```python
from build123d import *

# Parameters (mm, degrees)
ESQUISSE1_R                  = 11.15
BOSS_EXTRU_1_DEPTH           = 2
BOSS_EXTRU_2_DEPTH           = 80
BOSS_EXTRU_3_DEPTH           = 2.3
ENL_V_MAT_EXTRU_1_DEPTH      = 106.452595985
ENL_V_MAT_EXTRU_1_DEPTH_BACK = 106.452595985
ESQUISSE4_R                  = 1.55
BOSS_EXTRU_4_DEPTH           = 2
ENL_V_MAT_EXTRU_2_DEPTH      = 10
CONG_1_R                     = 2


with BuildPart() as part:
    # Esquisse1 → Boss.-Extru.1 (new body)
    with BuildSketch(Plane.XY):
        Polygon((-24.325901808, 28), (24.325901808, 28), (28, 24.325901808), (28, -24.325901808), (24.325901808, -28), (-24.325901808, -28), (-28, -24.325901808), (-28, 24.325901808), align=None)
        Circle(ESQUISSE1_R, mode=Mode.SUBTRACT)
    extrude(amount=BOSS_EXTRU_1_DEPTH)

    # Esquisse2 → Boss.-Extru.2 (add)
    with BuildSketch(Plane.XY.offset(2)):
        Polygon((-28, 24.325901808), (-28, -24.325901808), (-24.325901808, -28), (24.325901808, -28), (28, -24.325901808), (28, 24.325901808), (24.325901808, 28), (-24.325901808, 28), align=None)
        Polygon((-26.5, 23.704581464), (-26.5, -23.704581464), (-23.704581464, -26.5), (23.704581464, -26.5), (26.5, -23.704581464), (26.5, 23.704581464), (23.704581464, 26.5), (-23.704581464, 26.5), align=None, mode=Mode.SUBTRACT)
    extrude(amount=BOSS_EXTRU_2_DEPTH)

    # Esquisse3 → Boss.-Extru.3 (add)
    with BuildSketch(Plane(origin=(0, 0, 0), x_dir=(-1, 0, 0), z_dir=(0, 0, -1))):
        Polygon((-28, -20), (-28, 20), (-35.5, 12.5), (-35.5, -12.5), align=None)
        Polygon((-31.75, 3.175426481), (-34.5, 1.58771324), (-34.5, -1.58771324), (-31.75, -3.175426481), (-29, -1.58771324), (-29, 1.58771324), align=None, mode=Mode.SUBTRACT)
    extrude(amount=-BOSS_EXTRU_3_DEPTH)

    # Esquisse4 → Enlèv. mat.-Extru.1 (cut, two sides: drawn at the far end of the back side and taken through both)
    with BuildSketch(Plane(origin=(0, 28, 0), x_dir=(1, 0, 0), z_dir=(0, 1, 0)).offset(-ENL_V_MAT_EXTRU_1_DEPTH_BACK)):
        with Locations((0, -76)):
            Circle(ESQUISSE4_R)
    extrude(amount=ENL_V_MAT_EXTRU_1_DEPTH + ENL_V_MAT_EXTRU_1_DEPTH_BACK, mode=Mode.SUBTRACT)

    # Esquisse5 → Boss.-Extru.4 (add)
    with BuildSketch(Plane.XY.offset(2)):
        Polygon((-10.828088474, -1.05), (-12.1, -1.05), (-12.1, 1.05), (-10.828088474, 1.05), (-9.6, 1.05), (-9.6, -1.05), align=None)
    extrude(amount=-BOSS_EXTRU_4_DEPTH)

    # Esquisse6 → Enlèv. mat.-Extru.2 (cut)
    with BuildSketch(Plane.XY.offset(2.3)):
        Polygon((28, -20), (35.5, -12.5), (35.5, 12.5), (28, 20), align=None)
    extrude(amount=-ENL_V_MAT_EXTRU_2_DEPTH, mode=Mode.SUBTRACT)

    # Congé1
    cong_1_edges = [part.edges().sort_by_distance(p)[0] for p in [
        (-23.704581464, -26.5, 42),
        (23.704581464, -26.5, 42),
        (26.5, -23.704581464, 42),
        (26.5, 23.704581464, 42),
        (23.704581464, 26.5, 42),
        (-23.704581464, 26.5, 42),
        (-26.5, 23.704581464, 42),
        (-26.5, -23.704581464, 42),
    ]]
    fillet(cong_1_edges, radius=CONG_1_R)


solid = part.part
```
Work out the finished part from the listing and answer in its coordinate system (mm). A direction names the side the tool comes from. Give positions to 0.01 mm unless a question says otherwise; leave off trailing zeros. Loops run counter-clockwise (first coordinate to the right, second up) from the corner with the lowest first, then second, coordinate; pieces in that order, holes last. Notation, with made-up numbers: (33.25, 75.5) -> (44.25, 75.5) arc R18 ccw to (44.25, 93.5) -> close; hole circle Ø11 at (-40, 23). An arc over 180 degrees is marked (long way). Put each result on its own line as item: value. Start each with the question number.
Item 1: The part is cut by section D-D (y = -2). Give the vertices of the cut face in (x, z).
Item 2: Find the intervals of material crossed by L1, parallel to X at y = -8, z = 62; L2, parallel to Z at x = 0, y = 27, in increasing order. Write a range as [from, to].
Item 3: This flat-tipped pin is pushed along its axis until it touches: P1, Ø8, axis at x = 17.5, y = 9.5, coming from the +Z side. Where does it stop, or does it pass through?
Item 4: The part is cut by section C-C (y = 18.5). Give the vertices of the cut face in (x, z).
Item 5: The part is cut by section A-A (x = 0). Give the vertices of the cut face in (y, z).
Item 6: The mould has two halves that part along Y. Classify faces 4 (the face through (0, 26.5, 41)), 5 (the face through (-26.5, 0, 41)), 6 (the face through (-28, 0, 40)), 7 (the face through (0, 28, 40)): released by +Y, released by -Y, zero draft, split by the parting line, or undercut.
Item 7: Which of the six approach directions +Z, -Z, +X, -X, +Y, -Y give full straight-line access (tool end or side, diameter ignored) to faces 1 (the face through (-9.6, 0, 1)), 2 (the face through (-26.137, 26.189, 40.426)), 3 (the face through (26.5, 0, 41))?
Answers below:
1. outline: (-28, 0) -> (-10.97, 0) -> (-10.97, 2) -> (-26.5, 2) -> (-26.5, 82) -> (-28, 82) -> close; (10.97, 0) -> (28, 0) -> (28, 82) -> (26.5, 82) -> (26.5, 2) -> (10.97, 2) -> close
2. L1: [-28, -26.5], [26.5, 28]
2. L2: [0, 74.45], [77.55, 82]
3. P1: z = 2
4. outline: (-28, 0) -> (28, 0) -> (28, 82) -> (26.5, 82) -> (26.5, 2) -> (-26.5, 2) -> (-26.5, 82) -> (-28, 82) -> close
5. outline: (-28, 0) -> (-11.15, 0) -> (-11.15, 2) -> (-26.5, 2) -> (-26.5, 74.45) -> (-28, 74.45) -> close; (-28, 77.55) -> (-26.5, 77.55) -> (-26.5, 82) -> (-28, 82) -> close; (11.15, 0) -> (28, 0) -> (28, 74.45) -> (26.5, 74.45) -> (26.5, 2) -> (11.15, 2) -> close; (26.5, 77.55) -> (28, 77.55) -> (28, 82) -> (26.5, 82) -> close
6. face 4: undercut
6. face 5: undercut
6. face 6: zero draft
6. face 7: released by +Y
7. face 1: +Z, -Z
7. face 2: +Z, -Z, -X, +Y
7. face 3: +Z
